from build123d import *

# Parameters (mm, degrees)
SKETCH1_W           = 2
SKETCH1_H           = 2
BOSS_EXTRUDE1_DEPTH = 10
SKETCH2_W           = 10
SKETCH2_H           = 2
BOSS_EXTRUDE2_DEPTH = 10
SKETCH3_W           = 6
SKETCH3_H           = 6
CUT_EXTRUDE1_DEPTH  = 21.712315177


with BuildPart() as part:
    # Sketch1 → Boss-Extrude1 (new body)
    with BuildSketch(Plane(origin=(0, 0, 0), x_dir=(1, 0, 0), z_dir=(0, 1, 0))):
        Rectangle(SKETCH1_W, SKETCH1_H)
    extrude(amount=BOSS_EXTRUDE1_DEPTH)

    # Sketch2 → Boss-Extrude2 (add)
    with BuildSketch(Plane(origin=(0, 10, 0), x_dir=(-1, 0, 0), z_dir=(0, 1, 0))):
        Rectangle(SKETCH2_W, SKETCH2_H)
    extrude(amount=BOSS_EXTRUDE2_DEPTH)

    # Sketch3 → Cut-Extrude1 (cut, through all)
    with BuildSketch(Plane.XY.offset(1)):
        with Locations((0, 15)):
            Rectangle(SKETCH3_W, SKETCH3_H)
    extrude(amount=-CUT_EXTRUDE1_DEPTH, mode=Mode.SUBTRACT)


solid = part.part
Build history of the part. All positions in model axes, mm. A direction names the side the tool comes from. Coordinates: 2 decimals unless noted, no trailing zeros. Write each loop counter-clockwise with the first axis right and the second up, starting at its lowest first coordinate (ties: lowest second). Pieces come first, ordered by that corner, then holes.
(1) Mould opens along X. For faces 5 (the flat face through (-3, 10, 0)), 6 (the flat face through (-3, 15, 0)), 7 (the flat face through (3, 15, 0)), 8 (the flat face through (5, 15, 0)) say: pulls with the +X half, pulls with the -X half, needs draft (parallel to the pull), parting line crosses it, or undercut.
(2) Cut at D-D on y = 4. List the corners of the cut face in (x, z).
(3) Cut at A-A on y = 15.5. List the corners of the cut face in (x, z).
(4) Drill centre lines: line 1 (X direction, y = 15.75, z = 0.2); line 2 (Y direction, x = -0.5, z = 0.75); line 3 (Y direction, x = 2.5, z = -0.3). Where is each one in solid material? Low to high.
(5) 3-axis set-ups, long thin cutter, end or side, ignore diameter. For faces 1 (the flat face through (-1, 5, 0)), 2 (the flat face through (1, 11, -1)), 3 (the flat face through (0, 18, 0)), 4 (the flat face through (3, 10, 0)): which of +Z, -Z, +X, -X, +Y, -Y reach the whole face in a straight line?
(6) Pin check, flat tip, straight feed: pin 1 Ø1 at (x, z) = (-3, 0) entering from -Y. Stop position of the tip, or through.
(7) Cut at C-C on z = 0.2. List the corners of the cut face in (x, y).
(8) Cut at B-B on x = -2. List the corners of the cut face in (y, z).
Working result:
1. face 5: needs draft
1. face 6: undercut
1. face 7: undercut
1. face 8: pulls with the +X half
2. outline: (-1, -1) - (1, -1) - (1, 1) - (-1, 1) - close
3. outline: (-5, -1) - (-3, -1) - (-3, 1) - (-5, 1) - close; (3, -1) - (5, -1) - (5, 1) - (3, 1) - close
4. line 1: x = -5 to -3, 3 to 5
4. line 2: y = 0 to 12, 18 to 20
4. line 3: y = 10 to 12, 18 to 20
5. face 1: +Z, -Z, -X, -Y
5. face 2: -Z, +X, -X, +Y, -Y
5. face 3: +Z, -Z
5. face 4: +Z, -Z, +X, -Y
6. pin 1: stops at y = 10
7. outline: (-5, 10) - (-1, 10) - (-1, 0) - (1, 0) - (1, 10) - (5, 10) - (5, 20) - (-5, 20) - close; hole (-3, 12) - (3, 12) - (3, 18) - (-3, 18) - close
8. outline: (10, -1) - (12, -1) - (12, 1) - (10, 1) - close; (18, -1) - (20, -1) - (20, 1) - (18, 1) - close
